Can you work these out from the model? Positions are in its coordinate system, mm. Give positions to 0.01 mm unless a question says otherwise; leave off trailing zeros. Write each loop counter-clockwise with the first axis right and the second up, starting at its lowest first coordinate (ties: lowest second). Pieces come first, ordered by that corner, then holes. Notation, with made-up numbers: (-5, 9) -> (43, 9) arc R8 ccw to (43, 18) -> close; hole circle Ø6 at (64.5, -26.75). An arc over 180 degrees is marked (long way). One line per item, written item: value.
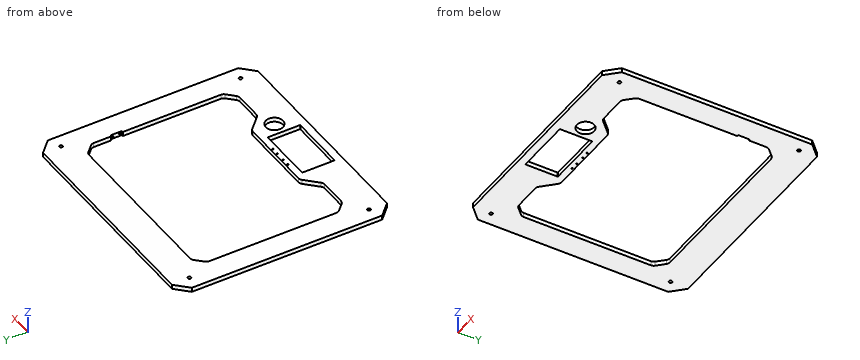
from build123d import *

# Parameters (mm, degrees)
BOSS_EXTRUDE1_DEPTH         = 9
CUT_EXTRUDE1_DEPTH          = 325.521282045
CUT_EXTRUDE2_DEPTH          = 325.521282045
SKETCH6_R                   = 17.5
CUT_EXTRUDE3_DEPTH          = 325.521282045
F_6_5_6_5_DIAMETER_HOLE1_D  = 6.5
CUT_EXTRUDE4_REACH          = 326.521
CUT_EXTRUDE5_REACH          = 326.521
SKETCH8_R                   = 1.25
CUT_EXTRUDE6_REACH          = 326.521
SKETCH9_W                   = 3
SKETCH9_H                   = 23.5
FILLET1_R                   = 0.5
M3_TAPPED_HOLE1_D           = 2.5
M3_TAPPED_HOLE1_DEPTH       = 10
M3_TAPPED_HOLE1_CSINK_D     = 3.05
M3_TAPPED_HOLE1_CSINK_ANGLE = 90
M3_TAPPED_HOLE1_TIP         = 0.751075774


with BuildPart() as part:
    # Sketch1 → Boss-Extrude1 (new body)
    with BuildSketch(Plane.XY):
        Polygon((-240, -193.25), (-215, -218.25), (215, -218.25), (240, -193.25), (240, 193.25), (215, 218.25), (-215, 218.25), (-240, 193.25), align=None)
    extrude(amount=-BOSS_EXTRUDE1_DEPTH)

    # Sketch2 → Cut-Extrude1 (cut, through all)
    with BuildSketch(Plane(origin=(0, 0, -9), x_dir=(-1, 0, 0), z_dir=(0, 0, -1))):
        with BuildLine():
            Line((114.142135624, -153.25), (168.357864376, -153.25))
            ThreePointArc((168.357864376, -153.25), (172.1846987, -152.488795325), (175.428932188, -150.321067812))
            Line((175.428932188, -150.321067812), (189.571067812, -136.178932188))
            ThreePointArc((189.571067812, -136.178932188), (191.738795325, -132.9346987), (192.5, -129.107864376))
            Line((192.5, -129.107864376), (192.5, 129.107864376))
            ThreePointArc((192.5, 129.107864376), (191.738795325, 132.9346987), (189.571067812, 136.178932188))
            Line((189.571067812, 136.178932188), (175.428932188, 150.321067812))
            ThreePointArc((175.428932188, 150.321067812), (172.1846987, 152.488795325), (168.357864376, 153.25))
            Line((168.357864376, 153.25), (-168.357864376, 153.25))
            ThreePointArc((-168.357864376, 153.25), (-172.1846987, 152.488795325), (-175.428932188, 150.321067812))
            Line((-175.428932188, 150.321067812), (-189.571067812, 136.178932188))
            ThreePointArc((-189.571067812, 136.178932188), (-191.738795325, 132.9346987), (-192.5, 129.107864376))
            Line((-192.5, 129.107864376), (-192.5, -129.107864376))
            ThreePointArc((-192.5, -129.107864376), (-191.738795325, -132.9346987), (-189.571067812, -136.178932188))
            Line((-189.571067812, -136.178932188), (-175.428932188, -150.321067812))
            ThreePointArc((-175.428932188, -150.321067812), (-172.1846987, -152.488795325), (-168.357864376, -153.25))
            Line((-168.357864376, -153.25), (-114.142135624, -153.25))
            ThreePointArc((-114.142135624, -153.25), (-110.3153013, -152.488795325), (-107.071067812, -150.321067812))
            Line((-107.071067812, -150.321067812), (-82.928932183, -126.178932183))
            ThreePointArc((-82.928932183, -126.178932183), (-79.684698695, -124.01120467), (-75.857864371, -123.249999995))
            Line((-75.857864371, -123.249999995), (75.857864371, -123.249999995))
            ThreePointArc((75.857864371, -123.249999995), (79.684698695, -124.01120467), (82.928932183, -126.178932183))
            Line((82.928932183, -126.178932183), (107.071067812, -150.321067812))
            ThreePointArc((107.071067812, -150.321067812), (110.3153013, -152.488795325), (114.142135624, -153.25))
        make_face()
    extrude(amount=-CUT_EXTRUDE1_DEPTH, mode=Mode.SUBTRACT)

    # Sketch3 → Cut-Extrude2 (cut, through all)
    with BuildSketch(Plane(origin=(0, 0, -9), x_dir=(-1, 0, 0), z_dir=(0, 0, -1))):
        with BuildLine():
            Line((48, -149.249999995), (-48, -149.249999995))
            ThreePointArc((-48, -149.249999995), (-48.707106781, -149.542893214), (-49, -150.249999995))
            Line((-49, -150.249999995), (-49, -189.249999995))
            ThreePointArc((-49, -189.249999995), (-48.707106781, -189.957106776), (-48, -190.249999995))
            Line((-48, -190.249999995), (48, -190.249999995))
            ThreePointArc((48, -190.249999995), (48.707106781, -189.957106776), (49, -189.249999995))
            Line((49, -189.249999995), (49, -150.249999995))
            ThreePointArc((49, -150.249999995), (48.707106781, -149.542893214), (48, -149.249999995))
        make_face()
    extrude(amount=-CUT_EXTRUDE2_DEPTH, mode=Mode.SUBTRACT)

    # Sketch6 → Cut-Extrude3 (cut, through all)
    with BuildSketch(Plane(origin=(0, 0, -9), x_dir=(-1, 0, 0), z_dir=(0, 0, -1))):
        with Locations(Location((-74.9, -166.249999995, 0), (0, 0, 180))):
            Circle(SKETCH6_R)
    extrude(amount=-CUT_EXTRUDE3_DEPTH, mode=Mode.SUBTRACT)

    # Ø6.5 (6.5) Diameter Hole1 (through all)
    with Locations(Plane.XY):
        with Locations((214, -182.25), (-214, -182.25), (-214, 182.25), (214, 182.25)):
            Hole(F_6_5_6_5_DIAMETER_HOLE1_D / 2)

    # Sketch7 → Cut-Extrude4 (cut, up to next)
    with BuildSketch(Plane(origin=(0, 0, -9), x_dir=(-1, 0, 0), z_dir=(0, 0, -1)), mode=Mode.PRIVATE) as cut_extrude4_sk1:
        with BuildLine():
            Line((-48, -136.75), (65, -136.75))
            ThreePointArc((65, -136.75), (65.707106781, -137.042893219), (66, -137.75))
            Line((66, -137.75), (66, -201.75))
            ThreePointArc((66, -201.75), (65.707106781, -202.457106781), (65, -202.75))
            Line((65, -202.75), (-48, -202.75))
            ThreePointArc((-48, -202.75), (-48.707106781, -202.457106781), (-49, -201.75))
            Line((-49, -201.75), (-49, -137.75))
            ThreePointArc((-49, -137.75), (-48.707106781, -137.042893219), (-48, -136.75))
        make_face()
    cut_extrude4_tool1 = extrude(cut_extrude4_sk1.sketch, amount=-CUT_EXTRUDE4_REACH, mode=Mode.PRIVATE) & part.part
    add(cut_extrude4_tool1.solids().sort_by_distance((-8.5, -169.75, -9))[0], mode=Mode.SUBTRACT)

    # Sketch8 → Cut-Extrude5 (cut, up to next)
    with BuildSketch(Plane.XY, mode=Mode.PRIVATE) as cut_extrude5_sk1:
        with Locations((-33.5, -127.541900756)):
            Circle(SKETCH8_R)
    cut_extrude5_tool1 = extrude(cut_extrude5_sk1.sketch, amount=-CUT_EXTRUDE5_REACH, mode=Mode.PRIVATE) & part.part
    # Sketch8 → Cut-Extrude5 (cut, up to next)
    with BuildSketch(Plane.XY, mode=Mode.PRIVATE) as cut_extrude5_sk2:
        with Locations((-18.5, -127.541900756)):
            Circle(SKETCH8_R)
    cut_extrude5_tool2 = extrude(cut_extrude5_sk2.sketch, amount=-CUT_EXTRUDE5_REACH, mode=Mode.PRIVATE) & part.part
    # Sketch8 → Cut-Extrude5 (cut, up to next)
    with BuildSketch(Plane.XY, mode=Mode.PRIVATE) as cut_extrude5_sk3:
        with Locations((1.5, -127.541900756)):
            Circle(SKETCH8_R)
    cut_extrude5_tool3 = extrude(cut_extrude5_sk3.sketch, amount=-CUT_EXTRUDE5_REACH, mode=Mode.PRIVATE) & part.part
    # Sketch8 → Cut-Extrude5 (cut, up to next)
    with BuildSketch(Plane.XY, mode=Mode.PRIVATE) as cut_extrude5_sk4:
        with Locations((16.5, -127.541900756)):
            Circle(SKETCH8_R)
    cut_extrude5_tool4 = extrude(cut_extrude5_sk4.sketch, amount=-CUT_EXTRUDE5_REACH, mode=Mode.PRIVATE) & part.part
    add(cut_extrude5_tool1.solids().sort_by_distance((-33.5, -127.541901, 0))[0], mode=Mode.SUBTRACT)
    add(cut_extrude5_tool2.solids().sort_by_distance((-18.5, -127.541901, 0))[0], mode=Mode.SUBTRACT)
    add(cut_extrude5_tool3.solids().sort_by_distance((1.5, -127.541901, 0))[0], mode=Mode.SUBTRACT)
    add(cut_extrude5_tool4.solids().sort_by_distance((16.5, -127.541901, 0))[0], mode=Mode.SUBTRACT)

    # Sketch9 → Cut-Extrude6 (cut, up to next)
    with BuildSketch(Plane.XY, mode=Mode.PRIVATE) as cut_extrude6_sk1:
        with Locations((194, 81.5)):
            Rectangle(SKETCH9_W, SKETCH9_H)
    cut_extrude6_tool1 = extrude(cut_extrude6_sk1.sketch, amount=-CUT_EXTRUDE6_REACH, mode=Mode.PRIVATE) & part.part
    add(cut_extrude6_tool1.solids().sort_by_distance((194, 81.5, 0))[0], mode=Mode.SUBTRACT)

    # Fillet1
    fillet1_edges = [part.edges().sort_by_distance(p)[0] for p in [
        (192.5, 69.75, -4.5),
        (192.5, 93.25, -4.5),
        (195.5, 93.25, -4.5),
        (195.5, 69.75, -4.5),
    ]]
    fillet(fillet1_edges, radius=FILLET1_R)

    # M3 Tapped Hole1
    with Locations(Plane.ZY.offset(-195.5)):
        with Locations((-4.5, 88.625), (-4.5, 74.375)):
            CounterSinkHole(M3_TAPPED_HOLE1_D / 2, M3_TAPPED_HOLE1_CSINK_D / 2, depth=M3_TAPPED_HOLE1_DEPTH, counter_sink_angle=M3_TAPPED_HOLE1_CSINK_ANGLE)
            with Locations((0, 0, -(M3_TAPPED_HOLE1_DEPTH + M3_TAPPED_HOLE1_TIP / 2))):  # 118° drill point
                Cone(0, M3_TAPPED_HOLE1_D / 2, M3_TAPPED_HOLE1_TIP, mode=Mode.SUBTRACT)


solid = part.part
1) If we section it at A-A (y = -166.25): Write out the boundary of the cut face in (x, z).
Answer list:
outline: (-240, -9) -> (-66, -9) -> (-66, 0) -> (-240, 0) -> close; (49, -9) -> (57.4, -9) -> (57.4, 0) -> (49, 0) -> close; (92.4, -9) -> (240, -9) -> (240, 0) -> (92.4, 0) -> close
2) I need wall thicknesses on L1, parallel to Y at x = 42.5, z = -2.5; L2, parallel to Y at x = 1.5, z = -3.5; L3, parallel to X at y = 182.25, z = -2. Which ranges of each line are inside material? Lowest first, please.
Answer list:
L1: y = -218.25 to -202.75, -136.75 to -123.25, 153.25 to 218.25
L2: y = -218.25 to -202.75, -136.75 to -128.79, -126.29 to -123.25, 153.25 to 218.25
L3: x = -240 to -217.25, -210.75 to 210.75, 217.25 to 240
3) If we section it at C-C (y = 51): Write out the boundary of the cut face in (x, z).
Answer list:
outline: (-240, -9) -> (-192.5, -9) -> (-192.5, 0) -> (-240, 0) -> close; (192.5, -9) -> (240, -9) -> (240, 0) -> (192.5, 0) -> close
4) If we section it at B-B (x = 158.5): Write out the boundary of the cut face in (y, z).
Answer list:
outline: (-218.25, -9) -> (-153.25, -9) -> (-153.25, 0) -> (-218.25, 0) -> close; (153.25, -9) -> (218.25, -9) -> (218.25, 0) -> (153.25, 0) -> close
